Part model, mm, in its own coordinate system. Give positions to 0.01 mm unless a question says otherwise; leave off trailing zeros. Write each loop counter-clockwise with the first axis right and the second up, starting at its lowest first coordinate (ties: lowest second). Pieces come first, ordered by that corner, then holes. Notation, with made-up numbers: M -11.5,5.25 L 27.5,5.25 A20 ccw 27.5,22.25 Z; hole C 34.25,49.25 d2. An arc over 180 degrees is marked long. Write item = value, one per line. Start each with the question number.
from build123d import *

# Parameters (mm, degrees)
SKETCH1_R             = 2.1
SKETCH1_R_2           = 1.5
BOSS_EXTRUDE1_DEPTH   = 5
DELETEFACE1_OUTLINE_R = 2.1
DELETEFACE1_DEPTH     = 5


# Read off the part's stored shape, not the designer's step: DeleteFace1
with BuildPart() as part:
    # Sketch1 → Boss-Extrude1 (new body)
    with BuildSketch(Plane.XY.offset(5)):
        Polygon((-24.04163056, 24.04163056), (0, 0), (125, 0), (149.04163056, 24.04163056), (149.04163056, 109.04163056), (125, 133.083261121), (0, 133.083261121), (-24.04163056, 109.04163056), align=None)
        with Locations((118.731419269, 101.776120312)):
            Circle(SKETCH1_R, mode=Mode.SUBTRACT)
        with Locations((78.347048523, 57.984145877)):
            Circle(SKETCH1_R, mode=Mode.SUBTRACT)
        with Locations((53.279835174, 85.131070757)):
            Circle(SKETCH1_R, mode=Mode.SUBTRACT)
        with Locations((46.652951477, 57.984145877)):
            Circle(SKETCH1_R, mode=Mode.SUBTRACT)
        with Locations((6.268580731, 31.307140809)):
            Circle(SKETCH1_R, mode=Mode.SUBTRACT)
        with Locations((6.268580731, 101.776120312)):
            Circle(SKETCH1_R, mode=Mode.SUBTRACT)
        with Locations((71.720164826, 47.952190364)):
            Circle(SKETCH1_R, mode=Mode.SUBTRACT)
        with Locations((78.347048523, 75.099115243)):
            Circle(SKETCH1_R, mode=Mode.SUBTRACT)
        with Locations((112.104535572, 111.808075826)):
            Circle(SKETCH1_R, mode=Mode.SUBTRACT)
        with Locations((118.731419269, 31.307140809)):
            Circle(SKETCH1_R, mode=Mode.SUBTRACT)
        with Locations((46.652951477, 75.099115243)):
            Circle(SKETCH1_R, mode=Mode.SUBTRACT)
        with Locations((53.279835174, 47.952190364)):
            Circle(SKETCH1_R, mode=Mode.SUBTRACT)
        with Locations((12.895464428, 21.275185295)):
            Circle(SKETCH1_R, mode=Mode.SUBTRACT)
        with Locations((12.895464428, 111.808075826)):
            Circle(SKETCH1_R, mode=Mode.SUBTRACT)
        with Locations((112.104535572, 21.275185295)):
            Circle(SKETCH1_R, mode=Mode.SUBTRACT)
        with Locations((71.720164826, 85.131070757)):
            Circle(SKETCH1_R, mode=Mode.SUBTRACT)
        with Locations((144.041630486, 94.041630337)):
            Circle(SKETCH1_R_2, mode=Mode.SUBTRACT)
        with Locations((-19.041630486, 39.041630784)):
            Circle(SKETCH1_R_2, mode=Mode.SUBTRACT)
        with Locations((144.041630486, 39.041630784)):
            Circle(SKETCH1_R_2, mode=Mode.SUBTRACT)
        with Locations((15.000000224, 5.000000075)):
            Circle(SKETCH1_R_2, mode=Mode.SUBTRACT)
        with Locations((109.999999776, 5.000000075)):
            Circle(SKETCH1_R_2, mode=Mode.SUBTRACT)
        with Locations((109.999999776, 128.083261046)):
            Circle(SKETCH1_R_2, mode=Mode.SUBTRACT)
        with Locations((15.000000224, 128.083261046)):
            Circle(SKETCH1_R_2, mode=Mode.SUBTRACT)
        with Locations((-19.041630486, 94.041630337)):
            Circle(SKETCH1_R_2, mode=Mode.SUBTRACT)
        Polygon((4.803542307, 37.516408095), (41.516606622, 61.768230885), (54.744873598, 41.742923077), (18.031809283, 17.491100287), align=None, mode=Mode.SUBTRACT)
        Polygon((18.031809283, 115.592160833), (54.744873598, 91.340338044), (41.516606622, 71.315030236), (4.803542307, 95.566853025), align=None, mode=Mode.SUBTRACT)
        Polygon((70.255126402, 41.742923077), (83.483393378, 61.768230885), (120.196457693, 37.516408095), (106.968190717, 17.491100287), align=None, mode=Mode.SUBTRACT)
        Polygon((83.483393378, 71.315030236), (70.255126402, 91.340338044), (106.968190717, 115.592160833), (120.196457693, 95.566853025), align=None, mode=Mode.SUBTRACT)
    extrude(amount=-BOSS_EXTRUDE1_DEPTH)

    # DeleteFace1 outline → DeleteFace1 (add)
    with BuildSketch(Plane.XY):
        Polygon((41.516606622, 61.768230885), (4.803542307, 37.516408095), (18.031809283, 17.491100287), (54.744873598, 41.742923077), align=None)
        Polygon((54.744873598, 91.340338044), (18.031809283, 115.592160833), (4.803542307, 95.566853025), (41.516606622, 71.315030236), align=None)
        Polygon((83.483393378, 61.768230885), (70.255126402, 41.742923077), (106.968190717, 17.491100287), (120.196457693, 37.516408095), align=None)
        Polygon((70.255126402, 91.340338044), (83.483393378, 71.315030236), (120.196457693, 95.566853025), (106.968190717, 115.592160833), align=None)
        with Locations((118.731419269, 101.776120312)):
            Circle(DELETEFACE1_OUTLINE_R)
        with Locations((78.347048523, 57.984145877)):
            Circle(DELETEFACE1_OUTLINE_R)
        with Locations((53.279835174, 85.131070757)):
            Circle(DELETEFACE1_OUTLINE_R)
        with Locations((46.652951477, 57.984145877)):
            Circle(DELETEFACE1_OUTLINE_R)
        with Locations((6.268580731, 31.307140809)):
            Circle(DELETEFACE1_OUTLINE_R)
        with Locations((6.268580731, 101.776120312)):
            Circle(DELETEFACE1_OUTLINE_R)
        with Locations((71.720164826, 47.952190364)):
            Circle(DELETEFACE1_OUTLINE_R)
        with Locations((78.347048523, 75.099115243)):
            Circle(DELETEFACE1_OUTLINE_R)
        with Locations((112.104535572, 111.808075826)):
            Circle(DELETEFACE1_OUTLINE_R)
        with Locations((118.731419269, 31.307140809)):
            Circle(DELETEFACE1_OUTLINE_R)
        with Locations((46.652951477, 75.099115243)):
            Circle(DELETEFACE1_OUTLINE_R)
        with Locations((53.279835174, 47.952190364)):
            Circle(DELETEFACE1_OUTLINE_R)
        with Locations((12.895464428, 21.275185295)):
            Circle(DELETEFACE1_OUTLINE_R)
        with Locations((12.895464428, 111.808075826)):
            Circle(DELETEFACE1_OUTLINE_R)
        with Locations((112.104535572, 21.275185295)):
            Circle(DELETEFACE1_OUTLINE_R)
        with Locations((71.720164826, 85.131070757)):
            Circle(DELETEFACE1_OUTLINE_R)
    extrude(amount=DELETEFACE1_DEPTH)


solid = part.part
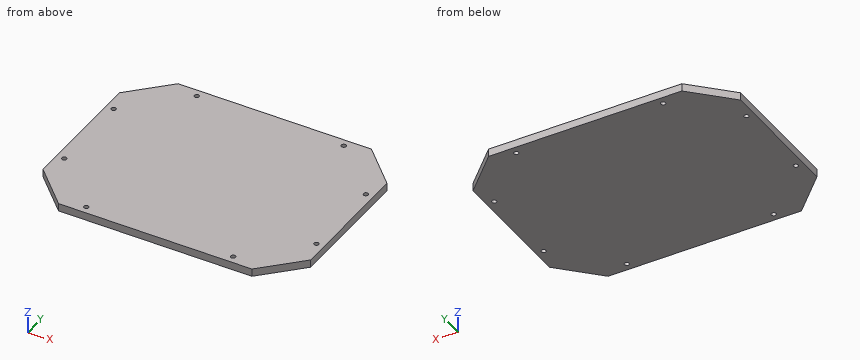
Q1. Slice it at A-A (z = 1.35). Give the number of separate pieces and of enclosed holes in the cut face, and give its area (3 significant figures).
Q2. Drop a flat-ended pin along its axis: P1, Ø1.8, axis at x = 110, y = 5, coming from the -Z side. Give the stop position or say it passes through.
Q3. Slice it at C-C (x = 133.5). Give the cut face in (y, z), and give its area (3 significant figures).
Q4. Probe line 1 along Y through (x, z) = (110, 1.3); line 2 along Y through (x, z) = (16, 4.05); line 3 along Y through (x, z) = (-6.5, 3.65). List the from-to ranges inside material, lowest first.
Q5. Slice it at B-B (y = 10). Give the cut face in (x, z), and give its area (3 significant figures).
Working result:
q1.separate_pieces = 1
q1.enclosed_holes = 8
q1.area = 21,800 mm2
q2.P1 = through
q3.outline = M 8.5,0 L 124.58,0 L 124.58,5 L 8.5,5 Z
q3.area = 580 mm2
q4.line_1 = 0 to 3.5, 6.5 to 126.58, 129.58 to 133.08
q4.line_2 = 0 to 3.88, 6.12 to 126.97, 129.2 to 133.08
q4.line_3 = 6.5 to 126.58
q5.outline = M -10,0 L 135,0 L 135,5 L -10,5 Z
q5.area = 725 mm2
